from build123d import *

# Parameters (mm, degrees)
SKETCH1_W           = 120
SKETCH1_H           = 100
BOSS_EXTRUDE1_DEPTH = 3
SKETCH2_R           = 2
CUT_EXTRUDE1_DEPTH  = 4
SKETCH3_R           = 2
CUT_EXTRUDE2_DEPTH  = 4
SKETCH4_R           = 2
CUT_EXTRUDE3_DEPTH  = 4


with BuildPart() as part:
    # Sketch1 → Boss-Extrude1 (new body)
    with BuildSketch(Plane(origin=(0, 0, 0), x_dir=(0, 0, -1), z_dir=(1, 0, 0))):
        with Locations((26.146465375, -0.01894847)):
            Rectangle(SKETCH1_W, SKETCH1_H)
    extrude(amount=BOSS_EXTRUDE1_DEPTH)

    # Sketch2 → Cut-Extrude1 (cut, through all)
    with BuildSketch(Plane(origin=(3, 0, 0), x_dir=(0, 0, -1), z_dir=(1, 0, 0))):
        with Locations((-3.853534625, -35.01894847)):
            Circle(SKETCH2_R)
        with Locations((56.146465375, -35.01894847)):
            Circle(SKETCH2_R)
    extrude(amount=-CUT_EXTRUDE1_DEPTH, mode=Mode.SUBTRACT)

    # Sketch3 → Cut-Extrude2 (cut, through all)
    with BuildSketch(Plane.ZY):
        with Locations((-68.146465375, -5.01894847)):
            Circle(SKETCH3_R)
        with Locations((15.853534625, -5.01894847)):
            Circle(SKETCH3_R)
    extrude(amount=-CUT_EXTRUDE2_DEPTH, mode=Mode.SUBTRACT)

    # Sketch4 → Cut-Extrude3 (cut, through all)
    with BuildSketch(Plane.ZY):
        with Locations((19.055575654, 34.98105153)):
            Circle(SKETCH4_R)
        with Locations((-71.348506404, 34.98105153)):
            Circle(SKETCH4_R)
    extrude(amount=-CUT_EXTRUDE3_DEPTH, mode=Mode.SUBTRACT)


solid = part.part
The model under review builds one solid part; all positions refer to its coordinate system, in mm. Coordinates: 2 decimals unless noted, no trailing zeros. Answer as CSV lines item,"result".
(1) For line 1 along Z through (x, y) = (1.1, -34); line 2 along Z through (x, y) = (2.45, -5.5); line 3 along Y through (x, z) = (2.1, 19), list the stretches that pass through material, from the lowest coordinate up. Write a range as [from, to].
Data:
line 1,"z = [-86.15, -57.87], [-54.43, 2.13], [5.57, 33.85]"
line 2,"z = [-86.15, -70.09], [-66.21, 13.91], [17.79, 33.85]"
line 3,"y = [-50.02, 32.98], [36.98, 49.98]"
(2) Mouldability with a two-part tool opening along Z and no side actions: class faces 1 (the cylindrical face through (1.521, -36.793, -57.069)), 2 (the flat face through (3, 1, -25)), 3 (the cylindrical face through (1.521, -36.793, 2.931)), 4 (the flat face through (1, -1, 33.854)) as pulls with the +Z half, pulls with the -Z half, needs draft (parallel to the pull), parting line crosses it, or undercut.
Data:
face 1,"undercut"
face 2,"needs draft"
face 3,"undercut"
face 4,"pulls with the +Z half"
(3) Clearance check with a flat-ended pin moving along its axis: pin 1 Ø5 at (y, z) = (34.98, -71.35) entering from +X. State where the tip first meets the part, or that it passes through.
Data:
pin 1,"stops at x = 3"
